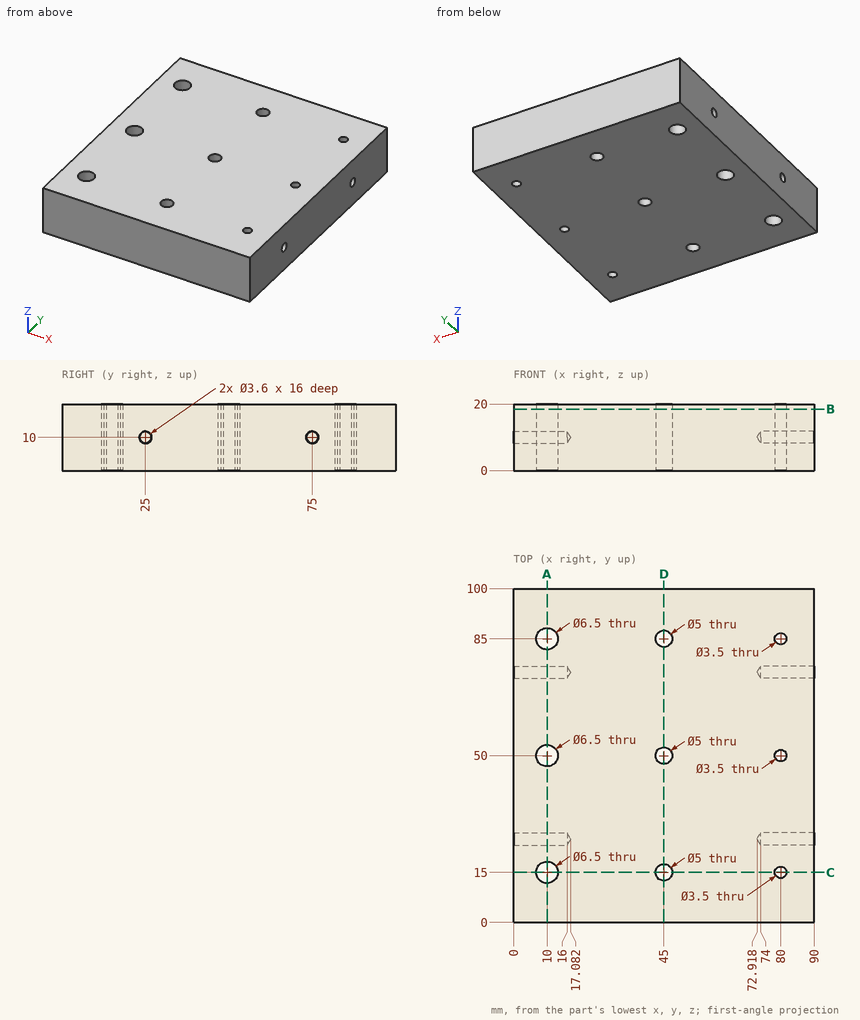
Check sheet for the drawn part. Datum: minimum x, y, z corner. Units: mm. Round coordinates to 2 decimals unless told otherwise and drop trailing zeros. Write each loop counter-clockwise with the first axis right and the second up, starting at its lowest first coordinate (ties: lowest second). Pieces come first, ordered by that corner, then holes. Notation, with made-up numbers: (18, 59.25) - (64, 59.25) arc R14 cw to (64, 68.25) - close; hole circle Ø9 at (1, -27). An arc over 180 degrees is marked (long way). Return JSON: item names as keys, results as strings.
Q1. Cross-section at B-B (z = 18.5). Give the number of separate pieces and of enclosed holes in the cut face, then the cut area to 3 significant figures.
Returned:
{"separate pieces": "1", "enclosed holes": "9", "area": "8,810 mm²"}
Q2. Cross-section at A-A (x = 10). Record the boundary of the cut face in (y, z), then the cut area to 3 significant figures.
Returned:
{"outline": "(0, 0) - (11.75, 0) - (11.75, 20) - (0, 20) - close; (18.25, 0) - (46.75, 0) - (46.75, 20) - (18.25, 20) - close; (53.25, 0) - (81.75, 0) - (81.75, 20) - (53.25, 20) - close; (88.25, 0) - (100, 0) - (100, 20) - (88.25, 20) - close; hole circle Ø3.6 at (25, 10); hole circle Ø3.6 at (75, 10)", "area": "1,590 mm²"}
Q3. Depth check by flat-ended pin: P1, Ø3, axis at x = 80, y = 15, coming from the +Z side; P2, Ø3, axis at y = 75, z = 10, coming from the +X side; P3, Ø3, axis at y = 75, z = 10, coming from the -X side. Enter the tip coordinate at first touch or a pass-through.
Returned:
{"P1": "passes through", "P2": "stops at x = 73.82", "P3": "stops at x = 16.18"}
Q4. Cross-section at D-D (x = 45). Record the boundary of the cut face in (y, z).
Returned:
{"outline": "(0, 0) - (12.5, 0) - (12.5, 20) - (0, 20) - close; (17.5, 0) - (47.5, 0) - (47.5, 20) - (17.5, 20) - close; (52.5, 0) - (82.5, 0) - (82.5, 20) - (52.5, 20) - close; (87.5, 0) - (100, 0) - (100, 20) - (87.5, 20) - close"}
Q5. Cross-section at C-C (y = 15). Record the boundary of the cut face in (x, z), then the cut area to 3 significant figures.
Returned:
{"outline": "(0, 0) - (6.75, 0) - (6.75, 20) - (0, 20) - close; (13.25, 0) - (42.5, 0) - (42.5, 20) - (13.25, 20) - close; (47.5, 0) - (78.25, 0) - (78.25, 20) - (47.5, 20) - close; (81.75, 0) - (90, 0) - (90, 20) - (81.75, 20) - close", "area": "1,500 mm²"}
Q6. Scan lines: L1, parallel to Y at x = 45, z = 7.75; L2, parallel to Y at x = 80, z = 14.5; L3, parallel to Y at x = 79.75, z = 10. Record each from-to range of solid material in increasing order. Write a range as from..to.
Returned:
{"L1": "y = 0..12.5, 17.5..47.5, 52.5..82.5, 87.5..100", "L2": "y = 0..13.25, 16.75..48.25, 51.75..83.25, 86.75..100", "L3": "y = 0..13.27, 16.73..23.2, 26.8..48.27, 51.73..73.2, 76.8..83.27, 86.73..100"}
